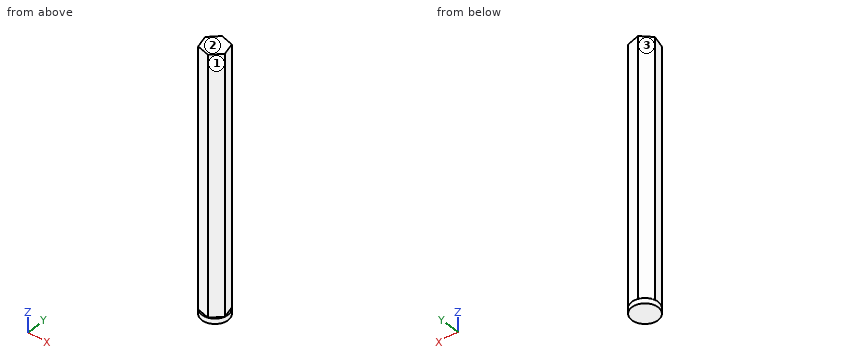
```python
from build123d import *

# Parameters (mm, degrees)
CROQUIS1_R              = 2.5
SALIENTE_EXTRUIR2_DEPTH = 1
SALIENTE_EXTRUIR3_DEPTH = 49


with BuildPart() as part:
    # Croquis1 → Saliente-Extruir2 (new body)
    with BuildSketch(Plane.XY):
        with Locations((-3.465701934, 4.477303942)):
            Circle(CROQUIS1_R)
    extrude(amount=SALIENTE_EXTRUIR2_DEPTH)

    # Croquis2 → Saliente-Extruir3 (add)
    with BuildSketch(Plane.XY.offset(1)):
        Polygon((-1.051265683, 3.828846087), (-1.696902833, 6.244038144), (-4.111339084, 6.892495999), (-5.880138185, 5.125761797), (-5.234501035, 2.71056974), (-2.820064784, 2.062111885), align=None)
    extrude(amount=SALIENTE_EXTRUIR3_DEPTH)


solid = part.part
```
Input: part model. Units: mm. Frame: model coordinates. Face numbers are marked on the shaded views. A direction names the side the tool comes from. Coordinates: 2 decimals unless noted, no trailing zeros. Write each loop counter-clockwise with the first axis right and the second up, starting at its lowest first coordinate (ties: lowest second). Pieces come first, ordered by that corner, then holes. Notation, with made-up numbers: M 35,63 L 61,63 A13 ccw 61,76 Z; hole C 4,-19.75 d8. An arc over 180 degrees is marked long. Use one line per item in the form item = value.
Q1. Set-up query: the marked faces 1, 2 and 3. Return all of +Z, -Z, +X, -X, +Y, -Y with unobstructed straight access to the full face (end or side cutting, diameter ignored); none if empty.
Answer below:
face_1 = +Z, +X, -Y
face_2 = +Z, +X, -X, +Y, -Y
face_3 = +Z, -X, +Y
Q2. Section A-A (z = 23). Return loops of the section in (x, y), plus the area to 3 significant figures.
Answer below:
outline = M -5.88,5.13 L -5.23,2.71 L -2.82,2.06 L -1.05,3.83 L -1.7,6.24 L -4.11,6.89 Z
area = 16.2 mm²
Q3. First-contact query: pin 1 (3 mm diameter, centred on x = -5, z = 39, fed in from +Y); pin 2 (1.5 mm diameter, centred on x = -3, z = 24.5, fed in from -Y); pin 3 (1.5 mm diameter, centred on y = 6, z = 28.5, fed in from -X). Flat tips, straight axial feed; report the tip coordinate or a pass-through.
Answer below:
pin_1 = 6.89
pin_2 = 2.06
pin_3 = -5.76
Q4. Section B-B (y = 5.6). Return loops of the section in (x, z).
Answer below:
outline = M -5.7,0 L -1.23,0 L -1.23,1 L -1.52,1 L -1.52,50 L -5.41,50 L -5.41,1 L -5.7,1 Z
Q5. Material intervals for probe 1 along Z at (x, y) = (-2.45, 6.6); probe 2 along Y at (x, z) = (-1.95, 47); probe 3 along Y at (x, z) = (-2.65, 45.5), sorted ascending. Write a range as from..to.
Answer below:
probe_1 = 0..1
probe_2 = 2.93..6.31
probe_3 = 2.23..6.5
Q6. Section C-C (x = -4.7). Return loops of the section in (y, z), plus the area to 3 significant figures.
Answer below:
outline = M 2.3,0 L 6.65,0 L 6.65,1 L 6.3,1 L 6.3,50 L 2.57,50 L 2.57,1 L 2.3,1 Z
area = 187 mm²
